```python
from build123d import *

# Parameters (mm, degrees)
SKETCH_1_W          = 60
SKETCH_1_H          = 128.259005876
EXTRUDE_1_DEPTH     = 3
SKETCH_2_R          = 4.5
CUT_EXTRUDE_1_DEPTH = 200.027899546
SKETCH_3_R          = 1.65
CUT_EXTRUDE_2_DEPTH = 200.027899546


with BuildPart() as part:
    # Эскиз1 → Бобышка-Вытянуть1 (new, symmetric)
    with BuildSketch(Plane(origin=(0, 0, 0), x_dir=(1, 0, 0), z_dir=(0, 1, 0))):
        with BuildLine():
            Line((-17.777747069, 78.129502938), (17.777747069, 78.129502938))
            Line((17.777747069, 78.129502938), (126.410491497, 117.062971345))
            ThreePointArc((126.410491497, 117.062971345), (150.551636651, 121.077456566), (130.031705733, 107.741662024))
            Line((130.031705733, 107.741662024), (40, 70))
            Line((40, 70), (40, -70))
            Line((40, -70), (130.031705733, -107.741662024))
            ThreePointArc((130.031705733, -107.741662024), (150.551636651, -121.077456566), (126.410491497, -117.062971345))
            Line((126.410491497, -117.062971345), (17.777747069, -78.129502938))
            Line((17.777747069, -78.129502938), (-17.777747069, -78.129502938))
            Line((-17.777747069, -78.129502938), (-126.410491497, -117.062971345))
            ThreePointArc((-126.410491497, -117.062971345), (-150.551636651, -121.077456566), (-130.031705733, -107.741662024))
            Line((-130.031705733, -107.741662024), (-40, -70))
            Line((-40, -70), (-40, 70))
            Line((-40, 70), (-130.031705733, 107.741662024))
            ThreePointArc((-130.031705733, 107.741662024), (-150.551636651, 121.077456566), (-126.410491497, 117.062971345))
            Line((-126.410491497, 117.062971345), (-17.777747069, 78.129502938))
        make_face()
        Rectangle(SKETCH_1_W, SKETCH_1_H, mode=Mode.SUBTRACT)
    extrude(amount=EXTRUDE_1_DEPTH, both=True)

    # Эскиз2 → Вырез-Вытянуть1 (cut, through all)
    with BuildSketch(Plane(origin=(0, 3, 0), x_dir=(1, 0, 0), z_dir=(0, 1, 0))):
        with Locations(Location((-138.9, 116.550938771, 0), (0, 0, 270))):
            Circle(SKETCH_2_R)
        with Locations(Location((138.9, 116.550938771, 0), (0, 0, 90))):
            Circle(SKETCH_2_R)
        with Locations(Location((138.9, -116.550938771, 0), (0, 0, 270))):
            Circle(SKETCH_2_R)
        with Locations(Location((-138.9, -116.550938771, 0), (0, 0, 90))):
            Circle(SKETCH_2_R)
        with BuildLine():
            ThreePointArc((-141.081727399, 125.151087929), (-143.394092115, 126.755135753), (-143.771780405, 123.966345414))
            ThreePointArc((-143.771780405, 123.966345414), (-141.459415689, 122.36229759), (-141.081727399, 125.151087929))
        make_face()
        with BuildLine():
            ThreePointArc((-130.299850841, 118.73266617), (-128.695803017, 121.045030885), (-131.484593356, 121.422719175))
            ThreePointArc((-131.484593356, 121.422719175), (-133.08864118, 119.110354459), (-130.299850841, 118.73266617))
        make_face()
        with BuildLine():
            ThreePointArc((-136.718272601, 107.950789612), (-134.405907885, 106.346741788), (-134.028219595, 109.135532127))
            ThreePointArc((-134.028219595, 109.135532127), (-136.340584311, 110.739579951), (-136.718272601, 107.950789612))
        make_face()
        with BuildLine():
            ThreePointArc((-147.500149159, 114.369211371), (-149.104196983, 112.056846656), (-146.315406644, 111.679158366))
            ThreePointArc((-146.315406644, 111.679158366), (-144.71135882, 113.991523082), (-147.500149159, 114.369211371))
        make_face()
        with BuildLine():
            ThreePointArc((146.315406644, 111.679158366), (144.71135882, 113.991523082), (147.500149159, 114.369211371))
            ThreePointArc((147.500149159, 114.369211371), (149.104196983, 112.056846656), (146.315406644, 111.679158366))
        make_face()
        with BuildLine():
            ThreePointArc((134.028219595, 109.135532127), (136.340584311, 110.739579951), (136.718272601, 107.950789612))
            ThreePointArc((136.718272601, 107.950789612), (134.405907885, 106.346741788), (134.028219595, 109.135532127))
        make_face()
        with BuildLine():
            ThreePointArc((131.484593356, 121.422719175), (133.08864118, 119.110354459), (130.299850841, 118.73266617))
            ThreePointArc((130.299850841, 118.73266617), (128.695803017, 121.045030885), (131.484593356, 121.422719175))
        make_face()
        with BuildLine():
            ThreePointArc((143.771780405, 123.966345414), (141.459415689, 122.36229759), (141.081727399, 125.151087929))
            ThreePointArc((141.081727399, 125.151087929), (143.394092115, 126.755135753), (143.771780405, 123.966345414))
        make_face()
        with BuildLine():
            ThreePointArc((141.081727399, -125.151087929), (143.394092115, -126.755135753), (143.771780405, -123.966345414))
            ThreePointArc((143.771780405, -123.966345414), (141.459415689, -122.36229759), (141.081727399, -125.151087929))
        make_face()
        with BuildLine():
            ThreePointArc((130.299850841, -118.73266617), (128.695803017, -121.045030885), (131.484593356, -121.422719175))
            ThreePointArc((131.484593356, -121.422719175), (133.08864118, -119.110354459), (130.299850841, -118.73266617))
        make_face()
        with BuildLine():
            ThreePointArc((136.718272601, -107.950789612), (134.405907885, -106.346741788), (134.028219595, -109.135532127))
            ThreePointArc((134.028219595, -109.135532127), (136.340584311, -110.739579951), (136.718272601, -107.950789612))
        make_face()
        with BuildLine():
            ThreePointArc((147.500149159, -114.369211371), (149.104196983, -112.056846656), (146.315406644, -111.679158366))
            ThreePointArc((146.315406644, -111.679158366), (144.71135882, -113.991523082), (147.500149159, -114.369211371))
        make_face()
        with BuildLine():
            ThreePointArc((-146.315406644, -111.679158366), (-144.71135882, -113.991523082), (-147.500149159, -114.369211371))
            ThreePointArc((-147.500149159, -114.369211371), (-149.104196983, -112.056846656), (-146.315406644, -111.679158366))
        make_face()
        with BuildLine():
            ThreePointArc((-134.028219595, -109.135532127), (-136.340584311, -110.739579951), (-136.718272601, -107.950789612))
            ThreePointArc((-136.718272601, -107.950789612), (-134.405907885, -106.346741788), (-134.028219595, -109.135532127))
        make_face()
        with BuildLine():
            ThreePointArc((-131.484593356, -121.422719175), (-133.08864118, -119.110354459), (-130.299850841, -118.73266617))
            ThreePointArc((-130.299850841, -118.73266617), (-128.695803017, -121.045030885), (-131.484593356, -121.422719175))
        make_face()
        with BuildLine():
            ThreePointArc((-143.771780405, -123.966345414), (-141.459415689, -122.36229759), (-141.081727399, -125.151087929))
            ThreePointArc((-141.081727399, -125.151087929), (-143.394092115, -126.755135753), (-143.771780405, -123.966345414))
        make_face()
    extrude(amount=-CUT_EXTRUDE_1_DEPTH, mode=Mode.SUBTRACT)

    # Эскиз3 → Вырез-Вытянуть2 (cut, through all)
    with BuildSketch(Plane(origin=(0, 3, 0), x_dir=(1, 0, 0), z_dir=(0, 1, 0))):
        with Locations(Location((-35, 76.19, 0), (0, 0, 270))):
            Circle(SKETCH_3_R)
        with Locations(Location((-35, 35, 0), (0, 0, 270))):
            Circle(SKETCH_3_R)
        with Locations(Location((-35, -35, 0), (0, 0, 90))):
            Circle(SKETCH_3_R)
        with Locations(Location((-35, -76.19, 0), (0, 0, 90))):
            Circle(SKETCH_3_R)
        with Locations(Location((35, -76.19, 0), (0, 0, 270))):
            Circle(SKETCH_3_R)
        with Locations(Location((35, -35, 0), (0, 0, 270))):
            Circle(SKETCH_3_R)
        with Locations(Location((35, 35, 0), (0, 0, 90))):
            Circle(SKETCH_3_R)
        with Locations(Location((35, 76.19, 0), (0, 0, 90))):
            Circle(SKETCH_3_R)
    extrude(amount=-CUT_EXTRUDE_2_DEPTH, mode=Mode.SUBTRACT)


solid = part.part
```
Geometry check sheet. Reference: the model listing, model coordinates, mm. A direction names the side the tool comes from. Round coordinates to 2 decimals unless told otherwise and drop trailing zeros. Loops run counter-clockwise (first coordinate to the right, second up) from the corner with the lowest first, then second, coordinate; pieces in that order, holes last. Notation, with made-up numbers: (4, 8) -> (8, 8) arc R26 cw to (8, 32) -> close; hole circle Ø1 at (38.5, 14). An arc over 180 degrees is marked (long way). Use a Markdown table: item, result.
(1) Go/stop test with flat-tipped pins: P1, Ø4, axis at x = 131.58, z = 119.78, coming from the -Y side; P2, Ø3, axis at y = 0.5, z = 1.5, coming from the -X side; P3, Ø1.5, axis at x = -41, y = 2, coming from the +Z side; P4, Ø1.5, axis at x = 68.5, y = -2, coming from the +Z side. Record where each tip stops, or that it passes through.
Calculated:
| item | result |
|---|---|
| P1 | y = -3 |
| P2 | x = -40 |
| P3 | z = 86.72 |
| P4 | z = 96.58 |
(2) Scan lines: probe 1 along Z at (x, y) = (-139, -2.6); probe 2 along X at (y, z) = (-2.55, 18.5); probe 3 along X at (y, z) = (-1.1, -76.19). Record each from-to range of solid material in increasing order.
Calculated:
| item | result |
|---|---|
| probe 1 | -129.05 to -121.05, -112.05 to -104.05, 104.05 to 112.05, 121.05 to 129.05 |
| probe 2 | -40 to -30, 30 to 40 |
| probe 3 | -54.77 to -36.65, -33.35 to 33.35, 36.65 to 54.77 |
(3) Sectioned sample at A-A (z = -8). Enter the section's corners in (x, y), then the cut area to 3 significant figures.
Calculated:
| item | result |
|---|---|
| outline | (-40, -3) -> (-30, -3) -> (-30, 3) -> (-40, 3) -> close; (30, -3) -> (40, -3) -> (40, 3) -> (30, 3) -> close |
| area | 120 mm² |
(4) Sectioned sample at B-B (x = -87). Enter the section's corners in (y, z), then the cut area to 3 significant figures.
Calculated:
| item | result |
|---|---|
| outline | (-3, -102.94) -> (3, -102.94) -> (3, -89.7) -> (-3, -89.7) -> close; (-3, 89.7) -> (3, 89.7) -> (3, 102.94) -> (-3, 102.94) -> close |
| area | 159 mm² |
(5) Mould release check, pull along X, two halves, no side actions. Record for faces 1 (the flat face through (-71.334, 0.042, 97.324)), 2 (the flat face through (40, 0, -1)), 3 (the flat face through (0, 0, -78.13)), 4 (the flat face through (-33, 3, -1)): released by +X, released by -X, zero draft, split by the parting line, or undercut.
Calculated:
| item | result |
|---|---|
| face 1 | undercut |
| face 2 | released by +X |
| face 3 | undercut |
| face 4 | zero draft |
(6) Set-up check for faces 5 (the flat face through (0, 0, -64.13)), 6 (the flat face through (-72.855, 0.042, -97.869)), 7 (the flat face through (72.855, 0.042, 97.869)): record each of +Z, -Z, +X, -X, +Y, -Y from which the full face is reachable in a straight line by a thin tool's end or side.
Calculated:
| item | result |
|---|---|
| face 5 | +Y, -Y |
| face 6 | -Z, +Y, -Y |
| face 7 | +Z, +Y, -Y |
